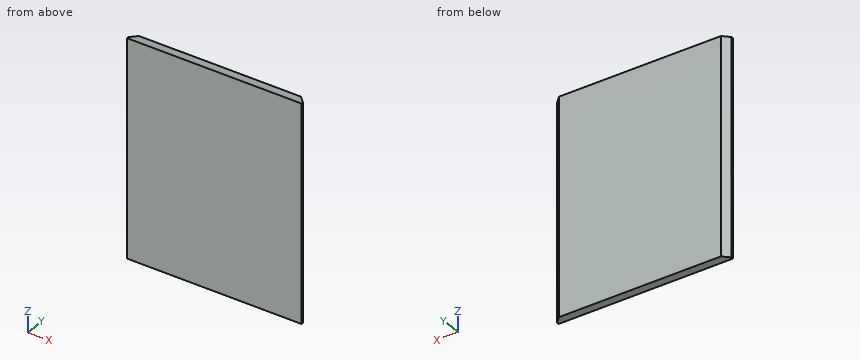
from build123d import *

# Parameters (mm, degrees)
SKETCH1_W           = 25.8
SKETCH1_H           = 2.65
BOSS_EXTRUDE1_DEPTH = 68.8


with BuildPart() as part:
    # Sketch1 → Boss-Extrude1 (new body)
    with BuildSketch(Plane.XY):
        Polygon((-2, 0.65), (-2, 0), (0, 0), (0, 2.65), align=None)
        with Locations((12.9, 1.325)):
            Rectangle(SKETCH1_W, SKETCH1_H)
    boss_extrude1 = extrude(amount=BOSS_EXTRUDE1_DEPTH)

    # Mirror1: Boss-Extrude1 across plane
    add(boss_extrude1.mirror(Plane(origin=(25.8, 0, 68.8), x_dir=(0, 0, 1), z_dir=(-1, 0, 0))))


solid = part.part
Geometry check sheet. Reference: the model listing, model coordinates, mm. Give positions to 0.01 mm unless a question says otherwise; leave off trailing zeros. Write each loop counter-clockwise with the first axis right and the second up, starting at its lowest first coordinate (ties: lowest second). Pieces come first, ordered by that corner, then holes.
1) Thickness scan on line 1 (X direction, y = 1.25, z = 59.5); line 2 (X direction, y = 1.35, z = 39.5). Record the ranges inside material, lowest first.
Values follow:
line 1: x = -1.4 to 53
line 2: x = -1.3 to 52.9
2) Cross-section at B-B (z = 15.5). Record the boundary of the cut face in (x, y), plus the area to 3 significant figures.
Values follow:
outline: (-2, 0) - (53.6, 0) - (53.6, 0.65) - (51.6, 2.65) - (0, 2.65) - (-2, 0.65) - close
area: 143 mm2
3) Cross-section at A-A (y = 2). Record the boundary of the cut face in (x, z).
Values follow:
outline: (-0.65, 0) - (52.25, 0) - (52.25, 68.8) - (-0.65, 68.8) - close
